The figure shows three views and two pictorial views of one solid part (mm, origin at its lowest corner). Answer the questions. Give positions to 0.01 mm unless a question says otherwise; leave off trailing zeros. Loops run counter-clockwise (first coordinate to the right, second up) from the corner with the lowest first, then second, coordinate; pieces in that order, holes last. Notation, with made-up numbers: (-32, 63) - (7, 63) arc R7 ccw to (7, 71) - close; hole circle Ø3 at (15, 29.25). An arc over 180 degrees is marked (long way). Write each question's results on one line, items separated by ' | '.
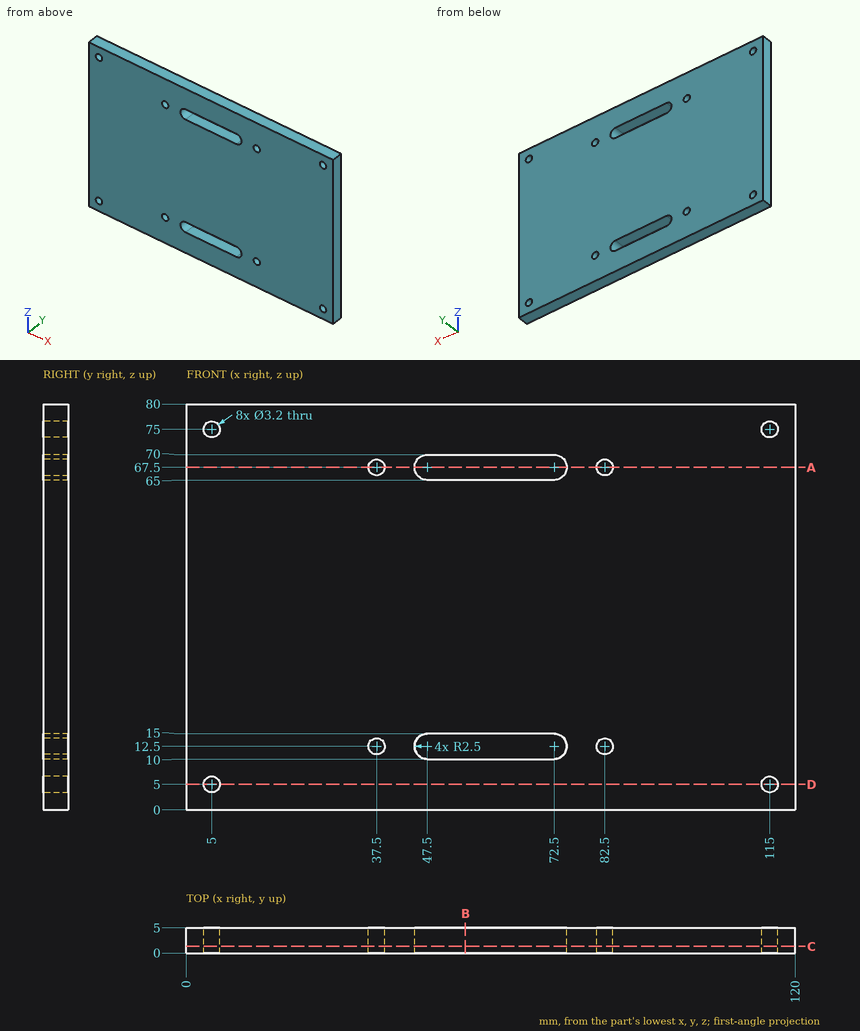
Item 1: A cutting plane is placed at C-C, the plane y = 1.35. Count the separate pieces of the cut face and the enclosed holes in it, plus the area to 3 significant figures.
Values found:
separate pieces: 1 | enclosed holes: 10 | area: 9,250 mm²
Item 2: A cutting plane is placed at B-B, the plane x = 55. Determine the outline of the cut face in (y, z), plus the area to 3 significant figures.
Values found:
outline: (0, 0) - (5, 0) - (5, 10) - (0, 10) - close; (0, 15) - (5, 15) - (5, 65) - (0, 65) - close; (0, 70) - (5, 70) - (5, 80) - (0, 80) - close | area: 350 mm²
Item 3: Find the intervals of material crossed by line 1 along Z through (x, y) = (55, 0.95); line 2 along X through (y, z) = (2.95, 12.5); line 3 along Z through (x, y) = (37.5, 2.1), in increasing order. Write a range as [from, to].
Values found:
line 1: z = [0, 10], [15, 65], [70, 80] | line 2: x = [0, 35.9], [39.1, 45], [75, 80.9], [84.1, 120] | line 3: z = [0, 10.9], [14.1, 65.9], [69.1, 80]
Item 4: A flat-ended cylindrical pin translates along its axis: P1, Ø3, axis at x = 5, z = 75, coming from the -Y side. Find the tip coordinate at first contact, or state that the pin passes through.
Values found:
P1: passes through
Item 5: A cutting plane is placed at A-A, the plane z = 67.5. Determine the outline of the cut face in (x, y), plus the area to 3 significant figures.
Values found:
outline: (0, 0) - (35.9, 0) - (35.9, 5) - (0, 5) - close; (39.1, 0) - (45, 0) - (45, 5) - (39.1, 5) - close; (75, 0) - (80.9, 0) - (80.9, 5) - (75, 5) - close; (84.1, 0) - (120, 0) - (120, 5) - (84.1, 5) - close | area: 418 mm²
Item 6: A cutting plane is placed at D-D, the plane z = 5. Determine the outline of the cut face in (x, y).
Values found:
outline: (0, 0) - (3.4, 0) - (3.4, 5) - (0, 5) - close; (6.6, 0) - (113.4, 0) - (113.4, 5) - (6.6, 5) - close; (116.6, 0) - (120, 0) - (120, 5) - (116.6, 5) - close
